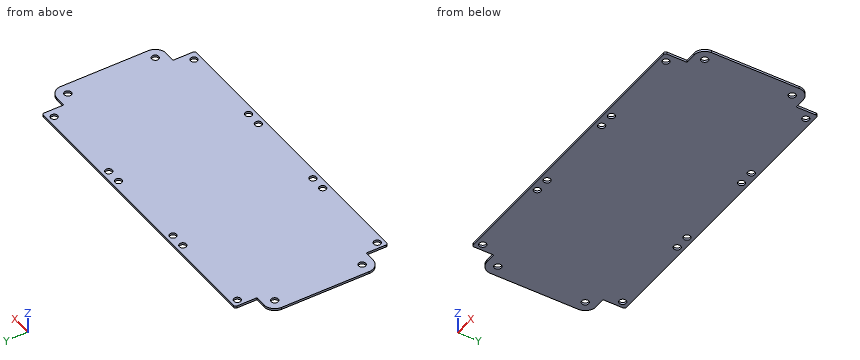
```python
from build123d import *

# Parameters (mm, degrees)
SKETCH1_R           = 1.6
BOSS_EXTRUDE1_DEPTH = 1


with BuildPart() as part:
    # Sketch1 → Boss-Extrude1 (new body)
    with BuildSketch(Plane.XY):
        with BuildLine():
            Line((110.085666764, -21.015048426), (110.085666764, -30.015048426))
            ThreePointArc((110.085666764, -30.015048426), (109.792773545, -30.722155207), (109.085666764, -31.015048426))
            Line((109.085666764, -31.015048426), (-26.914333236, -31.015048426))
            ThreePointArc((-26.914333236, -31.015048426), (-27.621440018, -30.722155207), (-27.914333236, -30.015048426))
            Line((-27.914333236, -30.015048426), (-27.914333236, -21.015048426))
            Line((-27.914333236, -21.015048426), (-32.914333236, -21.015048426))
            ThreePointArc((-32.914333236, -21.015048426), (-36.449867142, -19.550582332), (-37.914333236, -16.015048426))
            Line((-37.914333236, -16.015048426), (-37.914333236, 23.984951574))
            ThreePointArc((-37.914333236, 23.984951574), (-36.449867142, 27.52048548), (-32.914333236, 28.984951574))
            Line((-32.914333236, 28.984951574), (-27.914333236, 28.984951574))
            Line((-27.914333236, 28.984951574), (-27.914333236, 37.984951574))
            ThreePointArc((-27.914333236, 37.984951574), (-27.621440018, 38.692058356), (-26.914333236, 38.984951574))
            Line((-26.914333236, 38.984951574), (109.085666764, 38.984951574))
            ThreePointArc((109.085666764, 38.984951574), (109.792773545, 38.692058356), (110.085666764, 37.984951574))
            Line((110.085666764, 37.984951574), (110.085666764, 28.984951574))
            Line((110.085666764, 28.984951574), (115.085666764, 28.984951574))
            ThreePointArc((115.085666764, 28.984951574), (118.62120067, 27.52048548), (120.085666764, 23.984951574))
            Line((120.085666764, 23.984951574), (120.085666764, -16.015048426))
            ThreePointArc((120.085666764, -16.015048426), (118.62120067, -19.550582332), (115.085666764, -21.015048426))
            Line((115.085666764, -21.015048426), (110.085666764, -21.015048426))
        make_face()
        with Locations((-24.914333236, 35.984951574)):
            Circle(SKETCH1_R, mode=Mode.SUBTRACT)
        with Locations((14.085666764, 35.984951574)):
            Circle(SKETCH1_R, mode=Mode.SUBTRACT)
        with Locations((-24.914333236, -28.015048426)):
            Circle(SKETCH1_R, mode=Mode.SUBTRACT)
        with Locations((14.085666764, -28.015048426)):
            Circle(SKETCH1_R, mode=Mode.SUBTRACT)
        with Locations((21.085666764, 35.984951574)):
            Circle(SKETCH1_R, mode=Mode.SUBTRACT)
        with Locations((60.085666764, 35.984951574)):
            Circle(SKETCH1_R, mode=Mode.SUBTRACT)
        with Locations((60.085666764, -28.015048426)):
            Circle(SKETCH1_R, mode=Mode.SUBTRACT)
        with Locations((21.085666764, -28.015048426)):
            Circle(SKETCH1_R, mode=Mode.SUBTRACT)
        with Locations((67.085666764, 35.984951574)):
            Circle(SKETCH1_R, mode=Mode.SUBTRACT)
        with Locations((106.085666764, 35.984951574)):
            Circle(SKETCH1_R, mode=Mode.SUBTRACT)
        with Locations((106.085666764, -28.015048426)):
            Circle(SKETCH1_R, mode=Mode.SUBTRACT)
        with Locations((67.085666764, -28.015048426)):
            Circle(SKETCH1_R, mode=Mode.SUBTRACT)
        with Locations((-32.914333236, -16.015048426)):
            Circle(SKETCH1_R, mode=Mode.SUBTRACT)
        with Locations((-32.914333236, 23.984951574)):
            Circle(SKETCH1_R, mode=Mode.SUBTRACT)
        with Locations((115.085666764, 23.984951574)):
            Circle(SKETCH1_R, mode=Mode.SUBTRACT)
        with Locations((115.085666764, -16.015048426)):
            Circle(SKETCH1_R, mode=Mode.SUBTRACT)
    extrude(amount=BOSS_EXTRUDE1_DEPTH)


solid = part.part
```
Check sheet for the modelled part. Datum: model origin and axes. Units: mm. Give positions to 0.01 mm unless a question says otherwise; leave off trailing zeros. Use CSV: the item, a comma, the result in double quotes. Start each with the question number.
1) Material ranges on line 1 (Y direction, x = 15.5, z = 0.2); line 2 (Y direction, x = 14.5, z = 0.75); line 3 (Y direction, x = 111.5, z = 0.7), recorded low to high. Write a range as from..to.
2) Sectioned sample at A-A, the plane z = 0.5. Give the number of separate pieces and of enclosed holes in the cut face, plus the area to 3 significant figures.
3) Go/stop test with a flat-tipped pin: P1, Ø0.5, axis at y = 33, z = 0.5, coming from the +X side. Record where the tip stops, or that it passes through.
Recorded:
1,line 1,"-31.02..-28.76, -27.27..35.24, 36.73..38.98"
1,line 2,"-31.02..-29.56, -26.47..34.44, 37.53..38.98"
1,line 3,"-21.02..28.98"
2,separate pieces,"1"
2,enclosed holes,"16"
2,area,"10,500 mm2"
3,P1,"x = 110.09"
